from build123d import *

# Parameters (mm, degrees)
SKETCH3_R           = 0.7
BOSS_EXTRUDE1_DEPTH = 28.5
SKETCH4_R           = 1.25
BOSS_EXTRUDE3_DEPTH = 0.5


with BuildPart() as part:
    # Sketch1 → Revolve-Thin1 (revolve)
    with BuildSketch(Plane.XY):
        with BuildLine():
            ThreePointArc((0, -3.46), (3.46, 0), (0, 3.46))
            Line((0, 3.46), (0, 3.488))
            ThreePointArc((0, 3.488), (3.488, 0), (0, -3.488))
            Line((0, -3.488), (0, -3.46))
        make_face()
    revolve(axis=Axis((0, 3.46, 0), (0, -1, 0)))

    # Sketch3 → Boss-Extrude1 (add)
    with BuildSketch(Plane(origin=(0, 0, 0), x_dir=(1, 0, 0), z_dir=(0, 1, 0))):
        with Locations(Location((0, 0, 0), (0, 0, 90))):
            Circle(SKETCH3_R)
    extrude(amount=BOSS_EXTRUDE1_DEPTH)

    # Sketch4 → Boss-Extrude3 (add)
    with BuildSketch(Plane(origin=(0, 28.5, 0), x_dir=(1, 0, 0), z_dir=(0, 1, 0))):
        with Locations(Location((0, 0, 0), (0, 0, 270))):
            Circle(SKETCH4_R)
    extrude(amount=BOSS_EXTRUDE3_DEPTH)


solid = part.part
Input: part model. Units: mm. Frame: model coordinates. Round coordinates to 2 decimals unless told otherwise and drop trailing zeros. Order: outer loops, then holes, each group sorted by start corner. A loop starts at its lowest first (then second) coordinate and runs counter-clockwise, first axis right, second up. Notation, with made-up numbers: (-31, 2) - (14, 2) arc R24 ccw to (14, 12) - close; hole circle Ø8 at (-5.5, 57). An arc over 180 degrees is marked (long way). Answer as a JSON object with one key per item and string values. Group by question number.
(1) Material intervals for probe 1 along Z at (x, y) = (-0.5, 20); probe 2 along X at (y, z) = (11, -0.25), sorted ascending. Write a range as from..to.
(2) Cut plane B-B (z = 0). Return loops of the section in (x, y).
(3) Cut plane A-A (x = 0). Return loops of the section in (y, z), then the cut area to 3 significant figures.
(4) Pin query (flat end, axial travel): P1, Ø0.8, axis at x = 0, z = 0.5, coming from the -Y side; P2, Ø4, axis at x = -1, y = 14.5, coming from the -Z side; P3, Ø4, axis at x = -1, y = 19, coming from the +Z side. Return the tip coordinate at first contact, or that it passes through.
(5) Cut plane D-D (x = -2.5). Return loops of the section in (y, z), then the cut area to 3 significant figures.
(6) Cut plane C-C (y = 20). Return loops of the section in (x, z).
(7) Draft query along Y for faces 1 (the face through (-1.22, 28.75, -0.27)), 2 (the face through (0.683, 1.671, 0.152)), 3 (the face through (0, 29, 0)). Return one class per face: released by +Y, released by -Y, zero draft, split by the parting line, or undercut.
Here are the results:
{
 "1": {"probe 1": "z = -0.49..0.49", "probe 2": "x = -0.65..0.65"},
 "2": {"outline": "(-1.25, 28.5) - (-0.7, 28.5) - (-0.7, 3.42) arc R3.49 ccw (long way) to (0.7, 3.42) - (0.7, 28.5) - (1.25, 28.5) - (1.25, 29) - (-1.25, 29) - close; hole (-0.7, 0) - (-0.7, 3.39) arc R3.46 ccw (long way) to (0.7, 3.39) - (0.7, 0) - close"},
 "3": {"outline": "(3.42, -0.7) - (28.5, -0.7) - (28.5, -1.25) - (29, -1.25) - (29, 1.25) - (28.5, 1.25) - (28.5, 0.7) - (3.42, 0.7) arc R3.49 ccw (long way) to start; hole (0, -0.7) - (0, 0.7) - (3.39, 0.7) arc R3.46 ccw (long way) to (3.39, -0.7) - close", "area": "41.7 mm^2"},
 "4": {"P1": "stops at y = -3.49", "P2": "stops at z = -0.7", "P3": "stops at z = 0.7"},
 "5": {"outline": "circle Ø4.86 at (0, 0); hole circle Ø4.78 at (0, 0)", "area": "0.611 mm^2"},
 "6": {"outline": "circle Ø1.4 at (0, 0)"},
 "7": {"face 1": "zero draft", "face 2": "undercut", "face 3": "released by +Y"}
}
